Geometry check sheet. Reference: the model listing, model coordinates, mm. A direction names the side the tool comes from. Coordinates: 2 decimals unless noted, no trailing zeros. Order: outer loops, then holes, each group sorted by start corner. A loop starts at its lowest first (then second) coordinate and runs counter-clockwise, first axis right, second up.
```python
from build123d import *

# Parameters (mm, degrees)
SKETCH1_R           = 1.49999983
SKETCH1_R_2         = 1.50000021
BOSS_EXTRUDE5_DEPTH = 4


# Read off the part's stored shape, not the designer's step: Imported1
with BuildPart() as part:
    # Sketch1 → Boss-Extrude5 (new body)
    with BuildSketch(Plane.XY.offset(4.00000019)):
        with BuildLine():
            ThreePointArc((12.937500142, 43.342541903), (9.832499729, 46.447540761), (6.727500353, 43.342540866))
            Line((6.727500353, 43.342540866), (6.727500353, 23.671906441))
            ThreePointArc((6.727500353, 23.671906441), (0.018793936, 13.734902419), (7.902105327, 4.701398545))
            Line((7.902105327, 4.701398545), (7.524421789, 2.816406275))
            ThreePointArc((7.524421789, 2.816406275), (9.832500014, -5.9e-08), (12.14057824, 2.816406275))
            Line((12.14057824, 2.816406275), (11.762894778, 4.701398162))
            ThreePointArc((11.762894778, 4.701398162), (11.855672679, 5.730610746), (12.571502338, 6.475912151))
            ThreePointArc((12.571502338, 6.475912151), (12.653825046, 6.514541951), (12.738259166, 6.548308343))
            Line((12.738259166, 6.548308343), (13.279813023, 6.783419776))
            ThreePointArc((13.279813023, 6.783419776), (14.401344572, 6.854545961), (15.285156295, 6.160450299))
            Line((15.285156295, 6.160450299), (16.318864329, 4.609298912))
            ThreePointArc((16.318864329, 4.609298912), (19.954946163, 4.181790528), (19.61122341, 7.826747207))
            Line((19.61122341, 7.826747207), (18.012888788, 8.887330785))
            ThreePointArc((18.012888788, 8.887330785), (17.330815892, 9.745478763), (17.369938897, 10.840974441))
            Line((17.369938897, 10.840974441), (17.631297478, 11.478005982))
            ThreePointArc((17.631297478, 11.478005982), (18.378744789, 12.287790328), (19.473690584, 12.412377153))
            Line((19.473690584, 12.412377153), (21.358352668, 12.034519282))
            ThreePointArc((21.358352668, 12.034519282), (24.175042258, 14.342908104), (21.357632561, 16.650417974))
            Line((21.357632561, 16.650417974), (19.473808661, 16.272116711))
            ThreePointArc((19.473808661, 16.272116711), (19.473514795, 16.273584463), (19.473220705, 16.27505217))
            ThreePointArc((19.473220705, 16.27505217), (18.361090509, 16.40624384), (17.619571753, 17.245406971))
            Line((17.619571753, 17.245406971), (17.390357149, 17.796567545))
            ThreePointArc((17.390357149, 17.796567545), (17.322929979, 18.914964617), (18.012888788, 19.79775297))
            Line((18.012888788, 19.79775297), (19.611220282, 20.858331838))
            ThreePointArc((19.611220282, 20.858331838), (19.975539072, 24.482917782), (16.35037502, 24.124397156))
            Line((16.35037502, 24.124397156), (15.285156295, 22.524633456))
            ThreePointArc((15.285156295, 22.524633456), (15.284091495, 22.525342953), (15.283026603, 22.526052311))
            ThreePointArc((15.283026603, 22.526052311), (14.383790145, 21.826291172), (13.248170262, 21.919346761))
            Line((13.248170262, 21.919346761), (12.937500142, 22.051239386))
            Line((12.937500142, 22.051239386), (12.937500142, 23.67190695))
            Line((12.937500142, 23.67190695), (12.937500142, 43.342541903))
        make_face()
        with Locations((9.832499965, 14.342541504)):
            Circle(SKETCH1_R, mode=Mode.SUBTRACT)
        with Locations((9.832500097, 43.342539793)):
            Circle(SKETCH1_R_2, mode=Mode.SUBTRACT)
    extrude(amount=BOSS_EXTRUDE5_DEPTH)


solid = part.part
```
Item 1: Sectioned sample at A-A (x = 18.5). Record the cut outline in (y, z).
Item 2: Tool access check on faces 5 (the face through (18.8, 20.32, 5.97)), 6 (the face through (14.39, 6.86, 5.97)), 7 (the face through (15.8, 23.3, 6)), 8 (the face through (11.954, 3.746, 5.972)), 9 (the face through (7.716, 3.772, 5.972)). Record the directions out of +Z, -Z, +X, -X, +Y, -Y that give a thin tool (end or side, any length) a straight path to the whole face; none if there is none.
Item 3: Sectioned sample at B-B (z = 4.7). Give the number of separate pieces and of enclosed holes in the cut face, and give its area (3 significant figures).
Item 4: Sectioned sample at D-D (x = 9). Record the cut outline in (y, z).
Item 5: Release check for a two-part mould opening along Y. For faces 1 (the face through (20.429, 16.464, 5.972)), 2 (the face through (9.901, 46.447, 5.972)), 3 (the face through (20.403, 12.226, 5.972)), 4 (the face through (12, 18, 4)) record: pulls with the +Y half, pulls with the -Y half, needs draft (parallel to the pull), parting line crosses it, or undercut.
Item 6: Sectioned sample at C-C (y = 34.5). Record the cut outline in (x, z), and give its area (3 significant figures).
Item 7: Thickness scan on line 1 along Y through (x, z) = (20, 5.2); line 2 along X through (y, z) = (2.5, 7.65); line 3 along X through (y, z) = (34, 5.05). Record the ranges inside material, lowest first.
Geometry check:
1. outline: (3.52, 4) - (8.56, 4) - (8.56, 8) - (3.52, 8) - close; (12.34, 4) - (16.34, 4) - (16.34, 8) - (12.34, 8) - close; (20.12, 4) - (25.17, 4) - (25.17, 8) - (20.12, 8) - close
2. face 5: +Z, -Z, +X
2. face 6: +Z, -Z, -Y
2. face 7: +Z, -Z, +Y
2. face 8: +Z, -Z
2. face 9: +Z, -Z, -X
3. separate pieces: 1
3. enclosed holes: 2
3. area: 482 mm2
4. outline: (0.15, 4) - (13.09, 4) - (13.09, 8) - (0.15, 8) - close; (15.59, 4) - (42.09, 4) - (42.09, 8) - (15.59, 8) - close; (44.59, 4) - (46.33, 4) - (46.33, 8) - (44.59, 8) - close
5. face 1: undercut
5. face 2: pulls with the +Y half
5. face 3: undercut
5. face 4: needs draft
6. outline: (6.73, 4) - (12.94, 4) - (12.94, 8) - (6.73, 8) - close
6. area: 24.8 mm2
7. line 1: y = 4.23 to 7.5, 12.31 to 16.38, 21.18 to 24.46
7. line 2: x = 7.48 to 12.18
7. line 3: x = 6.73 to 12.94
